```python
from build123d import *

# Parameters (mm, degrees)
SKETCH11_W          = 10
SKETCH11_H          = 5
BOSS_EXTRUDE2_DEPTH = 8.5
SKETCH12_OUTSIDE_W  = 9.808
SKETCH12_OUTSIDE_H  = 13.308
CUT_EXTRUDE1_DEPTH  = 11
CUT_EXTRUDE2_DEPTH  = 8.3
CUT_EXTRUDE6_DEPTH  = 6
CUT_EXTRUDE3_DEPTH  = 1.5
CUT_EXTRUDE4_DEPTH  = 8.3
BOSS_EXTRUDE3_DEPTH = 9.5
CUT_EXTRUDE5_DEPTH  = 9.5
SKETCH19_R          = 0.5
CUT_EXTRUDE7_DEPTH  = 0.1
CUT_EXTRUDE8_START  = -0.1
SKETCH20_R          = 0.5
CUT_EXTRUDE8_DEPTH  = 0.1
SKETCH21_R          = 0.425
BOSS_EXTRUDE4_DEPTH = 1.2
SKETCH22_W          = 9.218939703
SKETCH22_H          = 4.445853418
BOSS_EXTRUDE5_DEPTH = 8.2
SKETCH23_W          = 12.5189076
SKETCH23_H          = 5
BOSS_EXTRUDE6_DEPTH = 0.3


with BuildPart() as part:
    # Sketch11 → Boss-Extrude2 (new body)
    with BuildSketch(Plane(origin=(0, 0, 0), x_dir=(1, 0, 0), z_dir=(0, 1, 0))):
        with Locations((5, 2.5)):
            Rectangle(SKETCH11_W, SKETCH11_H)
    extrude(amount=BOSS_EXTRUDE2_DEPTH)

    # Sketch12 outside → Cut-Extrude1 (cut)
    with BuildSketch(Plane(origin=(10, 0, 0), x_dir=(0, 0, -1), z_dir=(1, 0, 0))):
        with Locations((2.5, 4.25)):
            Rectangle(SKETCH12_OUTSIDE_W, SKETCH12_OUTSIDE_H)
        Polygon((0, 8.5), (0, 6.7), (0.2, 6.7), (0.2, 1.7), (0, 1.7), (0, 0), (5, 0), (5, 1.7), (4.8, 1.7), (4.8, 6.7), (5, 6.7), (5, 8.5), align=None, mode=Mode.SUBTRACT)
    extrude(amount=-CUT_EXTRUDE1_DEPTH, mode=Mode.SUBTRACT)

    # Sketch13 → Cut-Extrude2 (cut)
    with BuildSketch(Plane.XZ.offset(-8.5)):
        with BuildLine():
            Line((1, -0.6), (9, -0.6))
            ThreePointArc((9, -0.6), (9.141421356, -0.658578644), (9.2, -0.8))
            Line((9.2, -0.8), (9.2, -4.2))
            ThreePointArc((9.2, -4.2), (9.141421356, -4.341421356), (9, -4.4))
            Line((9, -4.4), (1, -4.4))
            ThreePointArc((1, -4.4), (0.858578644, -4.341421356), (0.8, -4.2))
            Line((0.8, -4.2), (0.8, -0.8))
            ThreePointArc((0.8, -0.8), (0.858578644, -0.658578644), (1, -0.6))
        make_face()
    extrude(amount=CUT_EXTRUDE2_DEPTH, mode=Mode.SUBTRACT)

    # Sketch18 → Cut-Extrude6 (cut)
    with BuildSketch(Plane(origin=(0, 8.5, 0), x_dir=(1, 0, 0), z_dir=(0, 1, 0))):
        with BuildLine():
            Line((1.5, 3.855615714), (4.2, 3.855615714))
            Line((4.2, 3.855615714), (4.2, 4.4))
            ThreePointArc((4.2, 4.4), (4.141421356, 4.541421356), (4, 4.6))
            Line((4, 4.6), (1.7, 4.6))
            ThreePointArc((1.7, 4.6), (1.558578644, 4.541421356), (1.5, 4.4))
            Line((1.5, 4.4), (1.5, 3.855615714))
        make_face()
    extrude(amount=-CUT_EXTRUDE6_DEPTH, mode=Mode.SUBTRACT)

    # Sketch14 → Cut-Extrude3 (cut)
    with BuildSketch(Plane.XZ.offset(-8.5)):
        with BuildLine():
            Line((8.5, -4.6), (1.5, -4.6))
            ThreePointArc((1.5, -4.6), (0.792893219, -4.307106781), (0.5, -3.6))
            Line((0.5, -3.6), (0.5, -1.4))
            ThreePointArc((0.5, -1.4), (0.792893219, -0.692893219), (1.5, -0.4))
            Line((1.5, -0.4), (8.5, -0.4))
            ThreePointArc((8.5, -0.4), (9.207106781, -0.692893219), (9.5, -1.4))
            Line((9.5, -1.4), (9.5, -3.6))
            ThreePointArc((9.5, -3.6), (9.207106781, -4.307106781), (8.5, -4.6))
        make_face()
    extrude(amount=CUT_EXTRUDE3_DEPTH, mode=Mode.SUBTRACT)

    # Sketch15 → Cut-Extrude4 (cut)
    with BuildSketch(Plane(origin=(0, 8.5, 0), x_dir=(1, 0, 0), z_dir=(0, 1, 0))):
        with BuildLine():
            Line((0.6, 3.6), (9.4, 3.6))
            ThreePointArc((9.4, 3.6), (9.470710678, 3.570710678), (9.5, 3.5))
            Line((9.5, 3.5), (9.5, 1.5))
            ThreePointArc((9.5, 1.5), (9.470710678, 1.429289322), (9.4, 1.4))
            Line((9.4, 1.4), (0.6, 1.4))
            ThreePointArc((0.6, 1.4), (0.529289322, 1.429289322), (0.5, 1.5))
            Line((0.5, 1.5), (0.5, 3.5))
            ThreePointArc((0.5, 3.5), (0.529289322, 3.570710678), (0.6, 3.6))
        make_face()
    extrude(amount=-CUT_EXTRUDE4_DEPTH, mode=Mode.SUBTRACT)

    # Sketch16 → Boss-Extrude3 (add)
    with BuildSketch(Plane.ZY):
        Polygon((-4.839479829, 0.939479829), (-4.1, 0.2), (-4.839479829, 0.2), align=None)
        Polygon((-0.9, 0.2), (-0.040645339, 1.059354661), (-0.040645339, 0.2), align=None)
    extrude(amount=-BOSS_EXTRUDE3_DEPTH)

    # Sketch17 → Cut-Extrude5 (cut)
    with BuildSketch(Plane(origin=(0, 8.5, 0), x_dir=(1, 0, 0), z_dir=(0, 1, 0))):
        Polygon((-0.242330702, 4.842330702), (0.3, 4.3), (-0.242330702, 3.757669298), align=None)
        Polygon((10.242330702, 3.757669298), (10.242330702, 4.842330702), (9.7, 4.3), align=None)
        Polygon((10.242330702, 0.157669298), (9.7, 0.7), (10.242330702, 1.242330702), align=None)
        Polygon((-0.242330702, 1.242330702), (-0.242330702, 0.157669298), (0.3, 0.7), align=None)
    extrude(amount=-CUT_EXTRUDE5_DEPTH, mode=Mode.SUBTRACT)

    # Sketch19 → Cut-Extrude7 (cut)
    with BuildSketch(Plane.XY):
        with Locations((0.9, 7.6)):
            Circle(SKETCH19_R)
    extrude(amount=-CUT_EXTRUDE7_DEPTH, mode=Mode.SUBTRACT)

    # Sketch20 → Cut-Extrude8 (cut)
    with BuildSketch(Plane(origin=(0, 0, -5), x_dir=(-1, 0, 0), z_dir=(0, 0, -1)).offset(CUT_EXTRUDE8_START)):
        with Locations(Location((-0.9, 7.6, 0), (0, 0, 180))):
            Circle(SKETCH20_R)
    extrude(amount=CUT_EXTRUDE8_DEPTH, mode=Mode.SUBTRACT)

    # Sketch21 → Boss-Extrude4 (add)
    with BuildSketch(Plane(origin=(0, 8.5, 0), x_dir=(1, 0, 0), z_dir=(0, 1, 0))):
        with BuildLine():
            Line((10.3, 3.55), (11.7, 3.55))
            Line((11.7, 3.55), (12, 3.25))
            Line((12, 3.25), (12, 1.75))
            Line((12, 1.75), (11.7, 1.45))
            Line((11.7, 1.45), (10.3, 1.45))
            ThreePointArc((10.3, 1.45), (10.087867966, 1.362132034), (10, 1.15))
            Line((10, 1.15), (10, 1))
            Line((10, 1), (9.555439603, 1))
            Line((9.555439603, 1), (9.555439603, 3.976356754))
            Line((9.555439603, 3.976356754), (10, 3.976356754))
            Line((10, 3.976356754), (10, 3.85))
            ThreePointArc((10, 3.85), (10.087867966, 3.637867966), (10.3, 3.55))
        make_face()
        with Locations(Location((11, 2.5, 0), (0, 0, 270))):
            Circle(SKETCH21_R, mode=Mode.SUBTRACT)
    extrude(amount=-BOSS_EXTRUDE4_DEPTH)

    # Sketch22 → Boss-Extrude5 (add)
    with BuildSketch(Plane(origin=(0, 0.2, 0), x_dir=(1, 0, 0), z_dir=(0, 1, 0))):
        with Locations((4.995733619, 2.483074162)):
            Rectangle(SKETCH22_W, SKETCH22_H)
    extrude(amount=BOSS_EXTRUDE5_DEPTH)

    # Sketch23 → Boss-Extrude6 (add)
    with BuildSketch(Plane(origin=(0, 8.5, 0), x_dir=(1, 0, 0), z_dir=(0, 1, 0))):
        with Locations((6.2594538, 2.5)):
            Rectangle(SKETCH23_W, SKETCH23_H)
    extrude(amount=BOSS_EXTRUDE6_DEPTH)


solid = part.part
```
Source: CAD feature listing. Evaluate the final solid. Frame: model axes, mm. A direction names the side the tool comes from. Coordinates: 2 decimals unless noted, no trailing zeros. Loops run counter-clockwise (first coordinate to the right, second up) from the corner with the lowest first, then second, coordinate; pieces in that order, holes last. Notation, with made-up numbers: M -20,-5 L 26,-5 A23 ccw 26,30 Z; hole C 68.5,35 d1. An arc over 180 degrees is marked long. Put each result on its own line as item: value. Start each with the question number.
1) Contact query for flat-ended pins moving along their axis: pin 1 Ø4 at (x, y) = (5.5, 4.5) entering from -Z; pin 2 Ø0.7 at (x, z) = (11, -2.5) entering from -Y; pin 3 Ø1.3 at (y, z) = (7.5, -2.5) entering from +X. Output: stop coordinate, or through.
2) Cut plane D-D on y = 0.75. Return the cut outline in (x, z), then the cut area to 3 significant figures.
3) Pull-direction query (Z, two-part tool) for faces 5 (the face through (0.9, 7.6, -0.1)), 6 (the face through (5, 8, -5)), 7 (the face through (11, 8.5, -2.5)); classes: pulls with the +Z half, pulls with the -Z half, needs draft (parallel to the pull), parting line crosses it, or undercut.
4) Ray query, L1, parallel to Z at x = 8, y = 3.75; L2, parallel to X at y = 7.7, z = -2.5 (3 decimals); L3, parallel to Y at x = 10.5, z = -3.2. Return the intervals inside material, ascending. Write a range as from..to.
5) Reachability of faces 1 (the face through (11, 8, -3.55)), 2 (the face through (5, 4, -4.8)), 3 (the face through (11, 8, -1.45)), 4 (the face through (5, 4, -0.2)) from +Z, -Z, +X, -X, +Y, -Y: full face, straight path, thin tool, end or side. Return the list, or none.
6) Cut plane C-C on x = 3. Return the cut outline in (y, z), then the cut area to 3 significant figures.
7) Cut plane A-A on z = -2.5. Return the cut outline in (x, y) (3 decimals).
The answers:
1. pin 1: stops at z = -4.8
1. pin 2: stops at y = 8.5
1. pin 3: stops at x = 12
2. outline: M 0,-5 L 10,-5 L 10,-4.6 L 9.7,-4.3 L 10,-4 L 10,-1 L 9.7,-0.7 L 10,-0.4 L 10,0 L 0,0 L 0,-0.4 L 0.3,-0.7 L 0,-1 L 0,-4 L 0.3,-4.3 L 0,-4.6 Z
2. area: 49.6 mm²
3. face 5: pulls with the +Z half
3. face 6: pulls with the -Z half
3. face 7: undercut
4. L1: z = -4.8..-0.2
4. L2: x = 0..10.575, 11.425..12
4. L3: y = 7.3..8.8
5. face 1: -Z, +X, -Y
5. face 2: -Z, +X, -X
5. face 3: +Z, +X, -Y
5. face 4: +Z, +X, -X
6. outline: M 0,-5 L 1.7,-5 L 1.7,-4.8 L 6.7,-4.8 L 6.7,-5 L 8.8,-5 L 8.8,0 L 6.7,0 L 6.7,-0.2 L 1.7,-0.2 L 1.7,0 L 0,0 Z; hole M 8.4,-4.6 L 8.5,-4.6 L 8.5,-0.4 L 8.4,-0.4 Z
6. area: 41.6 mm²
7. outline: M 0,0 L 10,0 L 10,7.3 L 10.575,7.3 L 10.575,8.5 L 11.425,8.5 L 11.425,7.3 L 12,7.3 L 12,8.5 L 12.519,8.5 L 12.519,8.8 L 0,8.8 Z; hole M 0.5,8.4 L 9.5,8.4 L 9.5,8.5 L 0.5,8.5 Z
